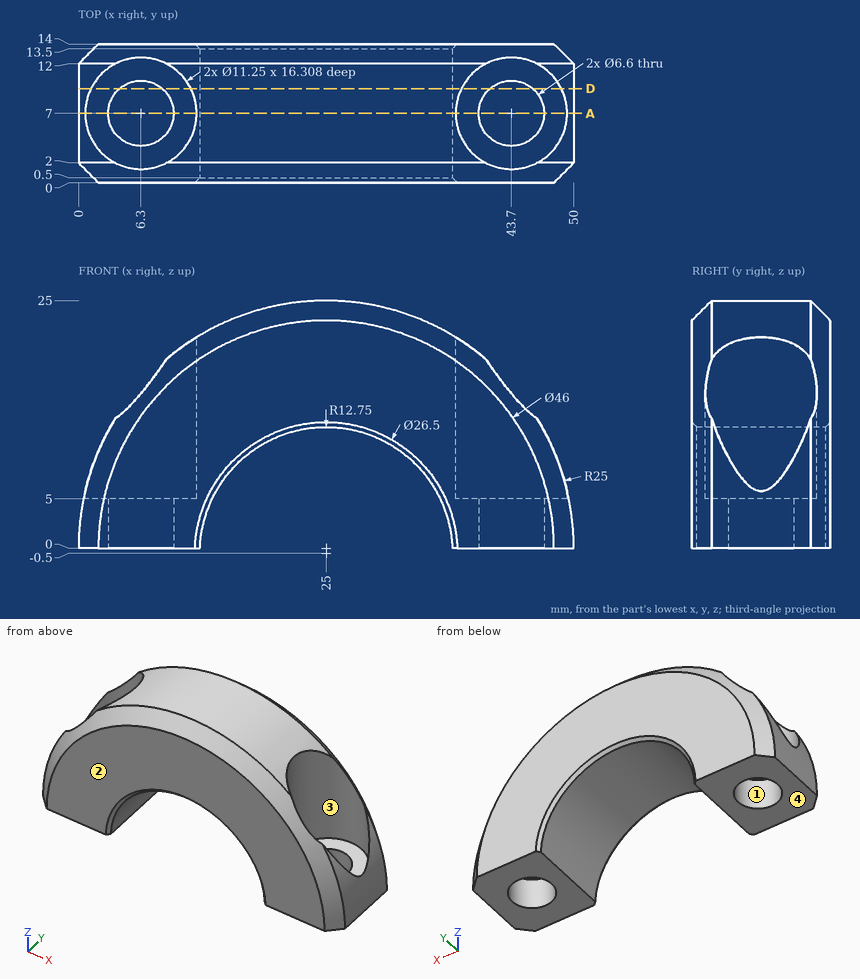
Could you check a few things on this drawing? It's one solid part, dimensions in mm from its lowest x, y, z. Coordinates: 2 decimals unless noted, no trailing zeros. Write each loop counter-clockwise with the first axis right and the second up, starting at its lowest first coordinate (ties: lowest second). Pieces come first, ordered by that corner, then holes.
1) If we section it at A-A (y = 7): Count the separate pieces of the cut face and the enclosed holes in it, plus the area to 3 significant figures.
Filled in:
separate pieces: 3
enclosed holes: 0
area: 432 mm2
2) I'm going to push flat-ended pins straight in: pin 1 (1.5 mm diameter, centred on y = 7, z = 11.5, fed in from -X) (1 decimal); pin 2 (6 mm diameter, centred on x = 39, y = 10.5, fed in from +Z); pin 3 (2 mm diameter, centred on x = 35, z = 6, fed in from -Y). Where does each tip first touch, or does it pass through?
Filled in:
pin 1: stops at x = 11.9
pin 2: stops at z = 22.45
pin 3: stops at y = 0.32
3) If I drill on line 1 (Y direction, x = 43.7, z = 2.5); line 2 (X direction, y = 7.75, z = 4.5); line 3 (Z direction, x = 48, y = 6), over which ranges is the centre line in solid material (lowest first)?
Filled in:
line 1: y = 0 to 3.7, 10.3 to 14
line 2: x = 0.41 to 3.09, 9.51 to 13.27, 36.73 to 40.49, 46.91 to 49.59
line 3: z = 0 to 5
4) Thinking about a two-plate mould opening in Y: for the marked faces 1, 2, 3 and 4, which applies, +Y half, -Y half, draft (parallel to the pull), parting line (faces both ways), or undercut?
Filled in:
face 1: undercut
face 2: -Y half
face 3: undercut
face 4: draft
5) If we section it at D-D (y = 9.5): List the corners of the cut face in (x, z) for me.
Filled in:
outline: (0, 0) - (4.15, 0) - (4.15, 5) - (1.26, 5) - (1.26, 7.84) arc R25 ccw to start; (8.45, 0) - (12.26, 0) arc R12.75 cw to (37.74, 0) - (41.55, 0) - (41.55, 5) - (38.66, 5) - (38.66, 20.94) arc R25 ccw to (11.34, 20.94) - (11.34, 5) - (8.45, 5) - close; (45.85, 0) - (50, 0) arc R25 ccw to (48.74, 7.84) - (48.74, 5) - (45.85, 5) - close
